```python
from build123d import *

# Parameters (mm, degrees)
BOSS_EXTRUDE1_DEPTH = 20
SKETCH2_R           = 2.75
CUT_EXTRUDE1_DEPTH  = 49.989794856
SKETCH3_R           = 2.75
CUT_EXTRUDE2_DEPTH  = 49.989794856


with BuildPart() as part:
    # Sketch1 → Boss-Extrude1 (new body)
    with BuildSketch(Plane.XY):
        Polygon((0, 0), (4, 0), (4, 36), (20, 36), (20, 40), (0, 40), align=None)
    extrude(amount=BOSS_EXTRUDE1_DEPTH)

    # Sketch2 → Cut-Extrude1 (cut, through all)
    with BuildSketch(Plane(origin=(0, 40, 0), x_dir=(1, 0, 0), z_dir=(0, 1, 0))):
        with Locations(Location((10, -10, 0), (0, 0, 270))):
            Circle(SKETCH2_R)
    extrude(amount=-CUT_EXTRUDE1_DEPTH, mode=Mode.SUBTRACT)

    # Sketch3 → Cut-Extrude2 (cut, through all)
    with BuildSketch(Plane.ZY):
        with Locations((10, 10)):
            Circle(SKETCH3_R)
        with Locations((10, 25)):
            Circle(SKETCH3_R)
    extrude(amount=-CUT_EXTRUDE2_DEPTH, mode=Mode.SUBTRACT)


solid = part.part
```
Geometry check sheet. Reference: the model listing, model coordinates, mm. A direction names the side the tool comes from. Coordinates: 2 decimals unless noted, no trailing zeros. Order: outer loops, then holes, each group sorted by start corner. A loop starts at its lowest first (then second) coordinate and runs counter-clockwise, first axis right, second up. Notation, with made-up numbers: M 32,-13.75 L 47,-13.75 A33 ccw 47,25.25 Z; hole C 72.5,54.5 d3. An arc over 180 degrees is marked long. Answer as a JSON object with one key per item and string values.
Q1. Tool access check on faces 1 (the flat face through (4, 18, 10)), 2 (the flat face through (20, 38, 10)). Record the directions out of +Z, -Z, +X, -X, +Y, -Y that give a thin tool (end or side, any length) a straight path to the whole face; none if there is none.
Results are:
{"face 1": "+Z, -Z, +X, -Y", "face 2": "+Z, -Z, +X, +Y, -Y"}
Q2. Release check for a two-part mould opening along Z. For faces 3 (the flat face through (3, 26, 0)), 4 (the flat face through (0, 20, 10)), 5 (the cylindrical face through (1.972, 27.727, 9.642)) record: released by +Z, released by -Z, zero draft, split by the parting line, or undercut.
Results are:
{"face 3": "released by -Z", "face 4": "zero draft", "face 5": "undercut"}
Q3. Cross-section at D-D on x = 2. Record the cut outline in (y, z).
Results are:
{"outline": "M 0,0 L 40,0 L 40,20 L 0,20 Z; hole C 10,10 d5.5; hole C 25,10 d5.5"}
Q4. Cross-section at B-B on z = 10. Record the cut outline in (x, y), and give its area (3 significant figures).
Results are:
{"outline": "M 0,0 L 4,0 L 4,7.25 L 0,7.25 Z; M 0,12.75 L 4,12.75 L 4,22.25 L 0,22.25 Z; M 0,27.75 L 4,27.75 L 4,36 L 7.25,36 L 7.25,40 L 0,40 Z; M 12.75,36 L 20,36 L 20,40 L 12.75,40 Z", "area": "158 mm²"}
Q5. Cross-section at A-A on y = 25. Record the cut outline in (x, z), and give its area (3 significant figures).
Results are:
{"outline": "M 0,0 L 4,0 L 4,7.25 L 0,7.25 Z; M 0,12.75 L 4,12.75 L 4,20 L 0,20 Z", "area": "58.0 mm²"}
Q6. Cross-section at C-C on x = 10. Record the cut outline in (y, z), and give its area (3 significant figures).
Results are:
{"outline": "M 36,0 L 40,0 L 40,7.25 L 36,7.25 Z; M 36,12.75 L 40,12.75 L 40,20 L 36,20 Z", "area": "58.0 mm²"}
Q7. Scan lines: line 1 (Y direction, x = 3, z = 10); line 2 (X direction, y = 38.1, z = 10); line 3 (Y direction, x = 12.25, z = 7.25). Record each from-to range of solid material in increasing order.
Results are:
{"line 1": "y = 0 to 7.25, 12.75 to 22.25, 27.75 to 40", "line 2": "x = 0 to 7.25, 12.75 to 20", "line 3": "y = 36 to 40"}
Q8. Depth check by flat-ended pin: pin 1 Ø6 at (y, z) = (20.5, 6) entering from +X; pin 2 Ø4.5 at (y, z) = (10, 10) entering from -X. Enter the tip coordinate at first touch or a pass-through.
Results are:
{"pin 1": "stops at x = 4", "pin 2": "passes through"}
